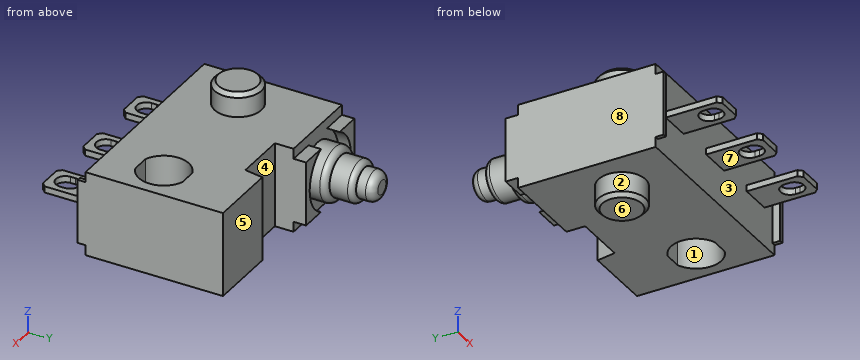
Autodesk Inventor part; units mm, degrees
ref_plane "YZ Plane" through (0, 0, 0) normal (1, 0, 0) x (0, 1, 0)
ref_plane "XZ Plane" through (0, 0, 0) normal (0, 1, 0) x (-1, 0, 0)
ref_plane "XY Plane" through (0, 0, 0) normal (0, 0, 1) x (1, 0, 0)
sketch "Skizze1" plane through (0, 0, 0) normal (0, 0, 1) x (1, 0, 0)
  line L0 (0, 0) -> (13.3, 0)
  line L1 (13.3, 0) -> (13.3, 8.8)
  line L2 (13.3, 8.8) -> (0, 8.8)
  line L3 (0, 8.8) -> (0, 0)
  circle A0 centre (2.7, 3.7) radius 1.5
  line L4 (0, 3.7) -> (13.3, 3.7) construction
  line L5 (10.4432, 5.2) -> (11.5568, 5.2)
  line L6 (10.4432, 2.2) -> (11.5568, 2.2)
  arc A1 (10.4432, 5.2) -> (10.4432, 2.2) centre (11, 3.7) ccw
  arc A2 (11.5568, 2.2) -> (11.5568, 5.2) centre (11, 3.7) ccw
  circle A3 centre (11, 3.7) radius 1.6 construction
  line L7 (1.12, 0) -> (3.12, 0)
  line L8 (3.12, 0) -> (3.12, -3.5)
  line L9 (3.12, -3.5) -> (1.12, -3.5)
  line L10 (1.12, -3.5) -> (1.12, 0)
  line L11 (5.65, 0) -> (7.65, 0)
  line L12 (7.65, 0) -> (7.65, -3.5)
  line L13 (7.65, -3.5) -> (5.65, -3.5)
  line L14 (5.65, -3.5) -> (5.65, 0)
  line L15 (10.18, 0) -> (12.18, 0)
  line L16 (12.18, 0) -> (12.18, -3.5)
  line L17 (12.18, -3.5) -> (10.18, -3.5)
  line L18 (10.18, -3.5) -> (10.18, 0)
  line L19 (0, 0) -> (0.25, 0)
  line L20 (0.25, 0) -> (0.25, -0.5)
  line L21 (0.25, -0.5) -> (0, -0.5)
  line L22 (0, -0.5) -> (0, 0)
  line L23 (13.3, 0) -> (13.05, 0)
  line L24 (13.05, 0) -> (13.05, -0.5)
  line L25 (13.05, -0.5) -> (13.3, -0.5)
  line L26 (13.3, -0.5) -> (13.3, 0)
  line L27 (2.12, 0) -> (2.12, -3.5) construction
  line L28 (6.65, 0) -> (6.65, -3.5) construction
  line L29 (11.18, 0) -> (11.18, -3.5) construction
  line L30 (11.18, -1.6) -> (11.18, -3.1) construction
  line L31 (10.58, -2.2) -> (10.58, -2.5)
  line L32 (11.78, -2.5) -> (11.78, -2.2)
  arc A4 (11.78, -2.2) -> (10.58, -2.2) centre (11.18, -2.2) ccw
  arc A5 (10.58, -2.5) -> (11.78, -2.5) centre (11.18, -2.5) ccw
  line L33 (2.12, -1.6) -> (2.12, -3.1) construction
  line L34 (1.52, -2.2) -> (1.52, -2.5)
  line L35 (2.72, -2.5) -> (2.72, -2.2)
  arc A6 (2.72, -2.2) -> (1.52, -2.2) centre (2.12, -2.2) ccw
  arc A7 (1.52, -2.5) -> (2.72, -2.5) centre (2.12, -2.5) ccw
  line L36 (6.65, -1.6) -> (6.65, -3.1) construction
  line L37 (6.05, -2.2) -> (6.05, -2.5)
  line L38 (7.25, -2.5) -> (7.25, -2.2)
  arc A8 (7.25, -2.2) -> (6.05, -2.2) centre (6.65, -2.2) ccw
  arc A9 (6.05, -2.5) -> (7.25, -2.5) centre (6.65, -2.5) ccw
  line L39 (5.4, 8.8) -> (5.4, 7.6)
  line L40 (5.4, 7.6) -> (8.7, 7.6)
  line L41 (8.7, 7.6) -> (8.9, 8.8)
  point P0 (13.175, -0.5)
  point P1 (11.18, -2.35)
  point P2 (2.12, -2.35)
  point P3 (6.65, -2.35)
  dimension "d0" = 13.3
  dimension "d3" = 3
  dimension "d4" = 3.7
  dimension "d5" = 5.1
  dimension "d6" = 3
  dimension "d7" = 2.7
  dimension "d8" = 8.3
  dimension "d10" = 3.2
  dimension "d11" = 4.2
  dimension "d12" = 0.25
  dimension "d13" = 0.25
  dimension "d14" = 4.53
  dimension "d15" = 4.53
  dimension "d16" = 2
  dimension "d17" = 3
  dimension "d18" = 1.5
  dimension "d19" = 1.2
  dimension "d23" = 1.5
  dimension "d24" = 1.2
  dimension "d25" = 0.4
  dimension "d26" = 0.4
  dimension "d27" = 1.5
  dimension "d28" = 1.2
  dimension "d29" = 0.4
  dimension "d30" = 5.4
  dimension "d32" = 3.3
  dimension "d33" = 1.2
  dimension "d34" = 3.5
extrude "Extrusion1" add sketch "Skizze1" along normal mid plane 5.4 contours L3 L2 L39 L40 L41 L1 L0
extrude "Extrusion2" add sketch "Skizze1" along normal mid plane 8.4 contours A0
extrude "Extrusion3" add sketch "Skizze1" along normal mid plane 0.4 contours L0 L8 L9 L10 | L0 L12 L13 L14 | L0 L16 L17 L18
extrude "Extrusion4" add sketch "Skizze1" along normal mid plane 4.1 contours L0 L20 L21 L22 | L26 L25 L24 L0
chamfer "Fase1" distance 0.25 angle 45 2 edges at (1.2, 3.7, 4.2) (1.2, 3.7, -4.2)
chamfer "Fase2" distance 0.25 angle 45 6 edges at (12.18, -3.5, 0) (10.18, -3.5, 0) (7.65, -3.5, 0) (5.65, -3.5, 0) (3.12, -3.5, 0) (1.12, -3.5, 0)
sketch "Skizze2" plane through (0, 8.8, 2.7) normal (0, 1, 0) x (1, 0, 0)
  line L0 (0, 5.4) -> (0, 0)
  line L1 (5.4, 0) -> (0, 0)
  line L2 (5.4, 5.4) -> (5.4, 0)
  line L3 (0, 5.4) -> (5.4, 5.4)
  circle A0 centre (2.7, 2.7) radius 2.7 construction
  circle A1 centre (2.7, 2.7) radius 1.7
  circle A2 centre (2.7, 2.7) radius 1.3
  circle A3 centre (2.7, 2.7) radius 0.95
  line L4 (5.4, 5.4) -> (5.4, 0)
  line L5 (0, 4.75) -> (5.4, 4.75)
  line L6 (5.4, 4.75) -> (5.4, 0.65)
  line L7 (5.4, 0.65) -> (0, 0.65)
  line L8 (0, 0.65) -> (0, 4.75)
  line L9 (0, 4.75) -> (5.4, 0.65) construction
  line L10 (5.4, 4.75) -> (0, 0.65) construction
  circle A4 centre (2.7, 2.7) radius 2.3
  point P0 (0, 2.7)
  point P1 (3.7428, 4.75)
  point P2 (3.7428, 0.65)
  point P3 (5.4, 0.65)
  point P4 (1.6572, 0.65)
  point P5 (1.6572, 4.75)
  dimension "d49" = 1.9
  dimension "d50" = 2.6
  dimension "d51" = 3.4
  dimension "d61" = 4.1
  dimension "d62" = 4.6
extrude "Extrusion5" add sketch "Skizze2" along normal blind 4.1 contours A3
extrude "Extrusion6" add sketch "Skizze2" along normal blind 3 contours A2
extrude "Extrusion7" add sketch "Skizze2" along normal blind 1.5 contours A1
fillet "Rundung1" radius 0.5 1 edges at (1.75, 12.9, 0)
fillet "Rundung2" radius 0.4 1 edges at (1, 10.3, 0)
fillet "Rundung3" radius 0.35 1 edges at (1.4, 11.8, 0)
extrude "Extrusion8" add sketch "Skizze2" along normal blind 0.8 contours L5 A4 L7 L0 | L2 L7 A4 L5
properties part number "Microswitch Panasonic" material "PVC, hart"
Design review of the part built by this model. Coordinates are the model's own, in mm. Face numbers are marked on the shaded views. A direction names the side the tool comes from. Coordinates: 2 decimals unless noted, no trailing zeros. Order: outer loops, then holes, each group sorted by start corner. A loop starts at its lowest first (then second) coordinate and runs counter-clockwise, first axis right, second up.
1) Take a section at C-C, the plane z = 0. State how many separate pieces and enclosed holes the cut face has, and give its area (3 significant figures).
2) Mouldability with a two-part tool opening along X and no side actions: class the marked faces 6, 7 and 8 as +X half, -X half, draft (parallel to the pull), parting line (faces both ways), or undercut.
3) Take a section at B-B, the plane z = -2.5. Give the boundary of the cut face in (x, y), and give its area (3 significant figures).
4) Wall thickness on line 1 along X through (y, z) = (9, -1.5); line 2 along Z through (x, y) = (1.5, -1); line 3 along Z through (x, y) = (4.5, 3.5): over which ranges is each line inside the solid? List them lowest first.
5) Take a section at D-D, the plane y = 5.5. Give the boundary of the cut face in (x, z).
6) For the marked faces 1, 2, 3, 4 and 5, list the 3-axis set-ups (+Z, -Z, +X, -X, +Y, -Y) from which the entire face can be reached by the end or side of a thin tool; tool diameter is ignored.
7) Clearance check with flat-ended pins moving along their axes: pin 1 (1.5 mm diameter, centred on y = 10, z = -1.5, fed in from +X); pin 2 (0.6 mm diameter, centred on x = 2.5, y = -1.5, fed in from -Z); pin 3 (0.5 mm diameter, centred on x = 1, z = 0.5, fed in from +Y). State where each tip first meets the part, or that it passes through.
8) Take a section at A-A, the plane y = 3.7. Give the boundary of the cut face in (x, z).
Returned:
1. separate pieces: 1
1. enclosed holes: 4
1. area: 133 mm2
2. face 6: draft
2. face 7: undercut
2. face 8: -X half
3. outline: (0, 0) - (13.3, 0) - (13.3, 8.8) - (8.9, 8.8) - (8.7, 7.6) - (5.4, 7.6) - (5.4, 8.8) - (0, 8.8) - close; hole (10.44, 2.2) - (11.56, 2.2) arc R1.6 ccw to (11.56, 5.2) - (10.44, 5.2) arc R1.6 ccw to start
3. area: 105 mm2
4. line 1: x = 0 to 0.96, 1.9 to 3.5, 4.44 to 5.4
4. line 2: z = -0.2 to 0.2
4. line 3: z = -2.7 to 2.7
5. outline: (0, -2.7) - (13.3, -2.7) - (13.3, 2.7) - (0, 2.7) - close
6. face 1: +Z, -Z
6. face 2: -Z
6. face 3: -Y
6. face 4: +Z, -Z, +Y
6. face 5: +Z, -Z, +X, +Y
7. pin 1: stops at x = 5.4
7. pin 2: stops at z = -0.2
7. pin 3: stops at y = 10.23
8. outline: (0, -2.7) - (1.2, -2.7) - (1.2, -3.95) - (1.45, -4.2) - (3.95, -4.2) - (4.2, -3.95) - (4.2, -2.7) - (9.4, -2.7) - (9.4, 2.7) - (4.2, 2.7) - (4.2, 3.95) - (3.95, 4.2) - (1.45, 4.2) - (1.2, 3.95) - (1.2, 2.7) - (0, 2.7) - close; (12.6, -2.7) - (13.3, -2.7) - (13.3, 2.7) - (12.6, 2.7) - close
